Check sheet for the drawn part. Datum: minimum x, y, z corner. Units: mm. A direction names the side the tool comes from. Round coordinates to 2 decimals unless told otherwise and drop trailing zeros. Order: outer loops, then holes, each group sorted by start corner. A loop starts at its lowest first (then second) coordinate and runs counter-clockwise, first axis right, second up.
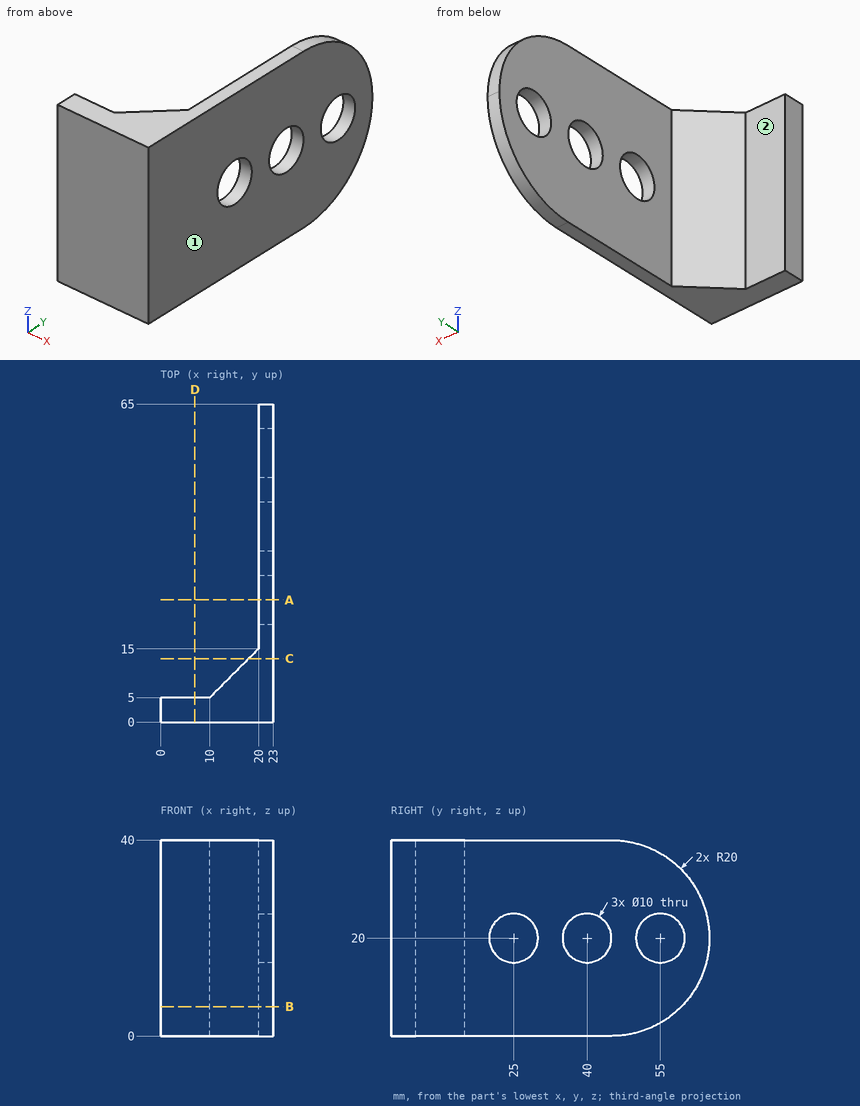
(1) Set-up check for the marked faces 1 and 2: record each of +Z, -Z, +X, -X, +Y, -Y from which the full face is reachable in a straight line by a thin tool's end or side.
Returned:
face 1: +Z, -Z, +X, +Y, -Y
face 2: +Z, -Z, -X, +Y
(2) Sectioned sample at C-C, the plane y = 13. Record the cut outline in (x, z), and give its area (3 significant figures).
Returned:
outline: (18, 0) - (23, 0) - (23, 40) - (18, 40) - close
area: 200 mm2
(3) Sectioned sample at B-B, the plane z = 6. Record the cut outline in (x, y).
Returned:
outline: (0, 0) - (23, 0) - (23, 59.28) - (20, 59.28) - (20, 15) - (10, 5) - (0, 5) - close
(4) Depth check by flat-ended pin: P1, Ø5, axis at y = 49, z = 20, coming from the -X side; P2, Ø5, axis at x = 5, z = 24, coming from the +Y side; P3, Ø6, axis at x = 19, z = 31, coming from the +Y side. Enter the tip coordinate at first touch or a pass-through.
Returned:
P1: stops at x = 20
P2: stops at y = 5
P3: stops at y = 63.25
(5) Sectioned sample at D-D, the plane x = 7. Record the cut outline in (y, z), and give its area (3 significant figures).
Returned:
outline: (0, 0) - (5, 0) - (5, 40) - (0, 40) - close
area: 200 mm2
(6) Material ranges on line 1 (Y direction, x = 21.15, z = 20); line 2 (X direction, y = 21, z = 32); line 3 (Y direction, x = 8.25, z = 33.5), recorded low to high.
Returned:
line 1: y = 0 to 20, 30 to 35, 45 to 50, 60 to 65
line 2: x = 20 to 23
line 3: y = 0 to 5
(7) Sectioned sample at A-A, the plane y = 25. Record the cut outline in (x, z).
Returned:
outline: (20, 0) - (23, 0) - (23, 15) - (20, 15) - close; (20, 25) - (23, 25) - (23, 40) - (20, 40) - close
